Build history of the part. All positions in model axes, mm. Give positions to 0.01 mm unless a question says otherwise; leave off trailing zeros. Loops run counter-clockwise (first coordinate to the right, second up) from the corner with the lowest first, then second, coordinate; pieces in that order, holes last. Notation, with made-up numbers: M 15.5,-28 L 43.5,-28 A34 cw 43.5,10 Z; hole C 14.25,63.5 d6. An arc over 180 degrees is marked long. Answer as a JSON object with one key per item and string values. Group by question number.
1. Drop a flat-ended pin along its axis: pin 1 Ø1 at (x, z) = (-0.5, 1.5) entering from -Y. Give the stop position or say it passes through.
2. Slice it at B-B (z = -0.25). List the corners of the cut face in (x, y), then the cut area to 3 significant figures.
3. Slice it at A-A (x = 0). List the corners of the cut face in (y, z), then the cut area to 3 significant figures.
4. Drill centre lines: line 1 along X through (y, z) = (0.35, -11); line 2 along Y through (x, z) = (0, 8.25); line 3 along Y through (x, z) = (-0.65, 13.5). Where is each one in solid material? Low to high. Write a range as [from, to].
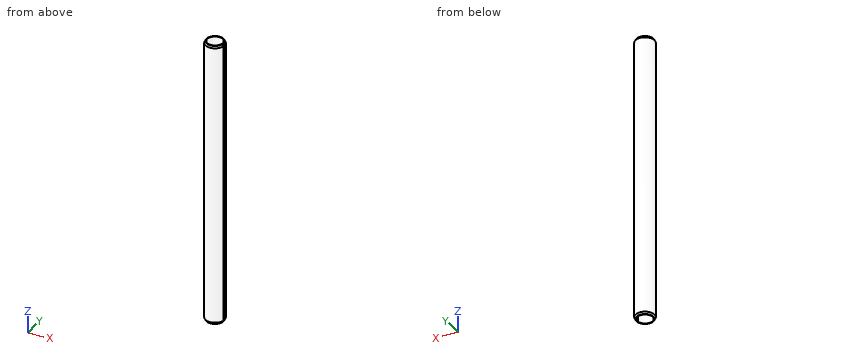
from build123d import *

# Parameters (mm, degrees)
REVOLVE1_ANGLE = 340


with BuildPart() as part:
    # Sketch2 → Revolve1 (revolve, symmetric)
    with BuildSketch(Plane(origin=(0, 0, 0), x_dir=(1, 0, 0), z_dir=(0, 1, 0))) as revolve1_sk:
        Polygon((-0.8, 15), (-0.9, 15), (-1, 14.8), (-1, -14.8), (-0.9, -15), (-0.8, -15), align=None)
    revolve(axis=Axis((0, 0, -15), (0, 0, 1)), revolution_arc=REVOLVE1_ANGLE / 2)
    revolve(revolve1_sk.sketch, axis=Axis((0, 0, -15), (0, 0, -1)), revolution_arc=REVOLVE1_ANGLE / 2)


solid = part.part
Established:
{
 "1": {"pin 1": "stops at y = -1"},
 "2": {"outline": "M 0.79,-0.14 A0.8 cw long 0.79,0.14 L 0.98,0.17 A1 ccw long 0.98,-0.17 Z", "area": "1.07 mm^2"},
 "3": {"outline": "M -1,-14.8 L -0.9,-15 L -0.8,-15 L -0.8,15 L -0.9,15 L -1,14.8 Z; M 0.8,-15 L 0.9,-15 L 1,-14.8 L 1,14.8 L 0.9,15 L 0.8,15 Z", "area": "12.0 mm^2"},
 "4": {"line 1": "x = [-0.94, -0.72], [0.72, 0.94]", "line 2": "y = [-1, -0.8], [0.8, 1]", "line 3": "y = [-0.76, -0.47], [0.47, 0.76]"}
}
